```python
from build123d import *

# Parameters (mm, degrees)
F1_DEPTH = 1
F2_DEPTH = 2
F3_W     = 13
F3_H     = 0.5
F4_DEPTH = 25.4
F5_SIZE  = 0.25
F6_R     = 0.3175


with BuildPart() as f1:
    # F0 (on Top) → F1 (new body)
    with BuildSketch(Plane.XY):
        with BuildLine():
            Line((13, -7.19), (13, 7.19))
            ThreePointArc((13, 7.19), (11.29829, 11.29829), (7.19, 13))
            Line((7.19, 13), (-7.19, 13))
            ThreePointArc((-7.19, 13), (-11.29829, 11.29829), (-13, 7.19))
            Line((-13, 7.19), (-13, -7.19))
            ThreePointArc((-13, -7.19), (-11.29829, -11.29829), (-7.19, -13))
            Line((-7.19, -13), (7.19, -13))
            ThreePointArc((7.19, -13), (11.29829, -11.29829), (13, -7.19))
        make_face()
        with BuildLine():
            ThreePointArc((-11, 7.19), (-9.884077, 9.884077), (-7.19, 11))
            Line((-7.19, 11), (7.19, 11))
            ThreePointArc((7.19, 11), (9.884077, 9.884077), (11, 7.19))
            Line((11, 7.19), (11, -7.19))
            ThreePointArc((11, -7.19), (9.884077, -9.884077), (7.19, -11))
            Line((7.19, -11), (-7.19, -11))
            ThreePointArc((-7.19, -11), (-9.884077, -9.884077), (-11, -7.19))
            Line((-11, -7.19), (-11, 7.19))
        make_face(mode=Mode.SUBTRACT)
    extrude(amount=F1_DEPTH)

    # F0 (on Top) → F2 (join)
    with BuildSketch(Plane.XY):
        with BuildLine():
            Line((7.19, 11), (-7.19, 11))
            ThreePointArc((-7.19, 11), (-9.884077, 9.884077), (-11, 7.19))
            Line((-11, 7.19), (-11, -7.19))
            ThreePointArc((-11, -7.19), (-9.884077, -9.884077), (-7.19, -11))
            Line((-7.19, -11), (7.19, -11))
            ThreePointArc((7.19, -11), (9.884077, -9.884077), (11, -7.19))
            Line((11, -7.19), (11, 7.19))
            ThreePointArc((11, 7.19), (9.884077, 9.884077), (7.19, 11))
        make_face()
    extrude(amount=F2_DEPTH)

    # F3 (on face) → F4 (cut)
    with BuildSketch(Plane.XY):
        with Locations((-6.5, -0.25)):
            Rectangle(F3_W, F3_H)
        with Locations((-6.5, 0.25)):
            Rectangle(F3_W, F3_H)
    extrude(amount=F4_DEPTH, mode=Mode.SUBTRACT)

    # F5
    f5_edges = [f1.edges().sort_by_distance(p)[0] for p in [
        (-11, -3.845, 2),
        (-11, 3.845, 2),
        (-9.884077, 9.884077, 2),
        (0, 11, 2),
        (11, 0, 2),
        (9.884077, -9.884077, 2),
        (0, -11, 2),
        (-9.884077, -9.884077, 2),
        (9.884077, 9.884077, 2),
    ]]
    chamfer(f5_edges, length=F5_SIZE)

    # F6
    f6_edges = [f1.edges().sort_by_distance(p)[0] for p in [
        (0, -0.5, 1),
        (0, 0.5, 1),
    ]]
    fillet(f6_edges, radius=F6_R)


solid = f1.part
```
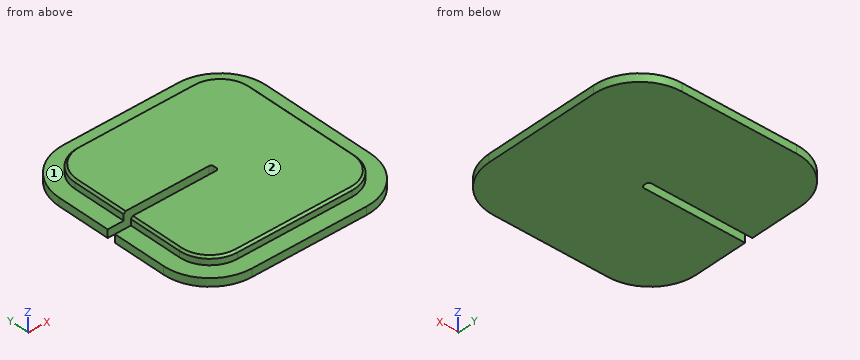
The model under review builds one solid part; all positions refer to its coordinate system, in mm. Face numbers are marked on the shaded views. A direction names the side the tool comes from. Coordinates: 2 decimals unless noted, no trailing zeros. Order: outer loops, then holes, each group sorted by start corner. A loop starts at its lowest first (then second) coordinate and runs counter-clockwise, first axis right, second up. Notation, with made-up numbers: M 9,-2.5 L 47,-2.5 A28 ccw 47,16.5 Z; hole C 87,-16 d1. An arc over 180 degrees is marked long. One line per question, with ' | ' between items.
(1) For probe 1 along Y at (x, z) = (-1, 1.1); probe 2 along Y at (x, z) = (-5.5, 0.15); probe 3 along X at (y, z) = (0.25, 0.2), list the stretches that pass through material, from the lowest coordinate up. Write a range as from..to.
Geometry results:
probe 1: y = -11..-0.5, 0.5..11 | probe 2: y = -13..-0.5, 0.5..13 | probe 3: x = -0.01..13
(2) Add section A-A, the plane x = -6.5. Write out the cut boundary in (y, z), then the cut area to 3 significant figures.
Geometry results:
outline: M -13,0 L -0.5,0 L -0.5,2 L -10.75,2 L -11,1.75 L -11,1 L -13,1 Z; M 0.5,0 L 13,0 L 13,1 L 11,1 L 11,1.75 L 10.75,2 L 0.5,2 Z | area: 45.9 mm²
(3) Add section B-B, the plane y = -4.25. Write out the cut boundary in (x, z).
Geometry results:
outline: M -13,0 L 13,0 L 13,1 L 11,1 L 11,1.75 L 10.75,2 L -10.75,2 L -11,1.75 L -11,1 L -13,1 Z
(4) Machinability: for the marked faces 1 and 2, which of the approach directions +Z, -Z, +X, -X, +Y, -Y give a long, thin tool a straight path to every point of the face, cutting with its end or side? Answer none if there is none.
Geometry results:
face 1: +Z | face 2: +Z, +X, -X, +Y, -Y
